For this review, take the finished solid that the model builds, in its own axes (mm). Face numbers are marked on the shaded views. A direction names the side the tool comes from. Round coordinates to 2 decimals unless told otherwise and drop trailing zeros. Order: outer loops, then holes, each group sorted by start corner. A loop starts at its lowest first (then second) coordinate and runs counter-clockwise, first axis right, second up. Notation, with made-up numbers: (5, 17) -> (40, 17) arc R5 cw to (40, 23) -> close; hole circle Ø1 at (-10.75, -24.5). An arc over 180 degrees is marked (long way). Use a Markdown table: item, result. Add a question column.
1) Wall thickness on line 1 along Z through (x, y) = (520, 1.5); line 2 along X through (y, z) = (16, 220.5); line 3 along Z through (x, y) = (-218.5, -16.5): over which ranges is each line inside the solid? List them lowest first. Write a range as [from, to].
2) Consider section B-B (x = -28.5). State the section outline as (y, z) points.
3) Machinability: for the marked faces 3 and 4, which of the approach directions +Z, -Z, +X, -X, +Y, -Y give a long, thin tool a straight path to every point of the face, cutting with its end or side? Answer none if there is none.
4) Consider section A-A (z = -439). State the section outline as (x, y) points.
5) Draft analysis for pull direction X (two halves, no side actions). For the marked faces 1 and 2, state which applies: pulls with the +X half, pulls with the -X half, needs draft (parallel to the pull), parting line crosses it, or undercut.
6) Clearance check with flat-ended pins moving along their axes: P1, Ø12, axis at y = 14.5, z = -365, coming from the -X side; P2, Ø10, axis at x = -48.5, z = -78, coming from the +Y side; P3, Ø20, axis at x = -7.5, y = 5, coming from the -Z side. State where each tip first meets the part, or that it passes through.
```python
from build123d import *

# Parameters (mm, degrees)
F1_DEPTH       = 20
F2_R           = 40
F3_DEPTH       = 50
F5_DEPTH       = 10
F7_DEPTH       = 10
F8_R           = 15
F9_DEPTH       = 80
F10_R          = 10
F11_DEPTH      = 100
F11_DEPTH_BACK = 100


with BuildPart() as f1:
    # F0 (on Front) → F1 (new body, symmetric)
    with BuildSketch(Plane.XZ):
        Polygon((600, 600), (-600, 600), (-600, 400), (-600, 180), (-600, -600), (600, -600), (600, 180), (600, 400), align=None)
        Polygon((-600, 180), (-600, 400), (-820, 260), (-820, 180), align=None)
        Polygon((820, 260), (600, 400), (600, 180), (820, 180), align=None)
    extrude(amount=F1_DEPTH, both=True)

    # F2 (on face) → F3 (cut)
    with BuildSketch(Plane.XZ.offset(20)):
        with Locations((-520, 520)):
            Circle(F2_R)
        with Locations((-520, -520)):
            Circle(F2_R)
        with Locations((520, 520)):
            Circle(F2_R)
        with Locations((520, -520)):
            Circle(F2_R)
    extrude(amount=-F3_DEPTH, mode=Mode.SUBTRACT)

    # F4 (on face) → F5 (cut)
    with BuildSketch(Plane.XZ.offset(20)):
        Polygon((360, 520), (-360, 520), (-520, 360), (-520, -360), (-360, -520), (360, -520), (520, -360), (520, 360), align=None)
    extrude(amount=-F5_DEPTH, mode=Mode.SUBTRACT)

    # F6 (on face) → F7 (cut)
    with BuildSketch(Plane(origin=(0, 20, 0), x_dir=(-1, 0, 0), z_dir=(0, 1, 0))):
        Polygon((360, -520), (520, -360), (520, 360), (360, 520), (-360, 520), (-520, 360), (-520, -360), (-360, -520), align=None)
    extrude(amount=-F7_DEPTH, mode=Mode.SUBTRACT)

    # F8 (on face) → F9 (join)
    with BuildSketch(Plane(origin=(-600, 0, 0), x_dir=(0, -1, 0), z_dir=(-1, 0, 0))):
        with Locations((0, -500)):
            Circle(F8_R)
    extrude(amount=F9_DEPTH)

    # F10 (on face) → F11 (join, two sides)
    with BuildSketch(Plane(origin=(0, 0, -600), x_dir=(1, 0, 0), z_dir=(0, 0, -1))) as f11_sk:
        with Locations((-670, 0)):
            Circle(F10_R)
    extrude(amount=-F11_DEPTH)
    extrude(f11_sk.sketch, amount=F11_DEPTH_BACK)


solid = f1.part
```
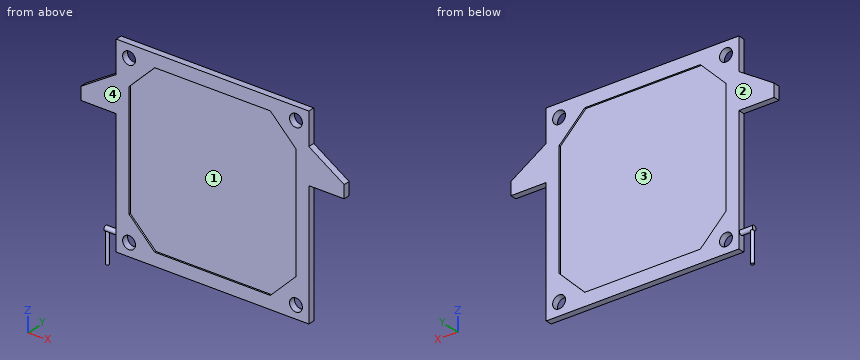
Results list:
| question | item | result |
|---|---|---|
| 1 | line 1 | [-600, -560], [-480, 480], [560, 600] |
| 1 | line 2 | [-820, -520], [520, 820] |
| 1 | line 3 | [-600, -520], [520, 600] |
| 2 | outline | (-20, -600) -> (20, -600) -> (20, -520) -> (10, -520) -> (10, 520) -> (20, 520) -> (20, 600) -> (-20, 600) -> (-20, 520) -> (-10, 520) -> (-10, -520) -> (-20, -520) -> close |
| 3 | face 3 | +Y |
| 3 | face 4 | +Z, -Z, +X, -X, -Y |
| 4 | outline | (-600, -20) -> (-441, -20) -> (-441, -10) -> (441, -10) -> (441, -20) -> (600, -20) -> (600, 20) -> (441, 20) -> (441, 10) -> (-441, 10) -> (-441, 20) -> (-600, 20) -> close |
| 5 | face 1 | undercut |
| 5 | face 2 | needs draft |
| 6 | P1 | x = -600 |
| 6 | P2 | y = 10 |
| 6 | P3 | z = -600 |
